```python
from build123d import *

# Parameters (mm, degrees)
F2_SIZE        = 1
F4_D           = 5
F4_DEPTH       = 15
F4_TIP         = 1.5021515476
F7_D           = 9
F7_DEPTH       = 6.3
F7_CSINK_D     = 17.92
F7_CSINK_ANGLE = 90
F7_TIP         = 2.7038727856


with BuildPart() as f1:
    # F0 (on Right) → F1 (revolve)
    with BuildSketch(Plane.YZ):
        Polygon((-17.5, 10), (-17.5, 0), (17.5, 0), (17.5, 10), (9.5, 10), (9.5, 12.5), (7.5, 12.5), (7.5, 10), align=None)
    revolve(axis=Axis((0, 0, 0), (0, 1, 0)))

    # F2
    f2_edges = [f1.edges().sort_by_distance(p)[0] for p in [
        (0, 17.5, -10),
        (0, -17.5, -10),
    ]]
    chamfer(f2_edges, length=F2_SIZE)

    # F4
    with Locations(Plane.XZ.offset(17.5)):
        with Locations((0, 0)):
            Hole(F4_D / 2, depth=F4_DEPTH)
            with Locations((0, 0, -(F4_DEPTH + F4_TIP / 2))):  # 118° drill point
                Cone(0, F4_D / 2, F4_TIP, mode=Mode.SUBTRACT)

    # F7
    with Locations(Plane.XZ.offset(20.5)):
        with Locations((0, 0)):
            CounterSinkHole(F7_D / 2, F7_CSINK_D / 2, depth=F7_DEPTH, counter_sink_angle=F7_CSINK_ANGLE)
            with Locations((0, 0, -(F7_DEPTH + F7_TIP / 2))):  # 118° drill point
                Cone(0, F7_D / 2, F7_TIP, mode=Mode.SUBTRACT)


solid = f1.part
```
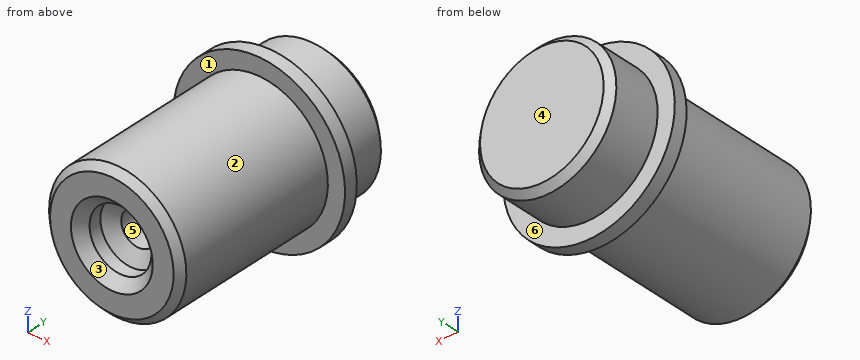
Design review of the part built by this model. Coordinates are the model's own, in mm. Face numbers are marked on the shaded views. A direction names the side the tool comes from. Coordinates: 2 decimals unless noted, no trailing zeros. Order: outer loops, then holes, each group sorted by start corner. A loop starts at its lowest first (then second) coordinate and runs counter-clockwise, first axis right, second up.
1) For the marked faces 4, 5 and 6, list the 3-axis set-ups (+Z, -Z, +X, -X, +Y, -Y) from which the entire face can be reached by the end or side of a thin tool; tool diameter is ignored.
2) Take a section at B-B, the plane y = 15.5. Give the boundary of the cut face in (x, z), and give its area (3 significant figures).
3) Clearance check with flat-ended pins moving along their axes: pin 1 (8 mm diameter, centred on x = 2.5, y = -4, fed in from -Z); pin 2 (2 mm diameter, centred on x = 6.5, z = 9, fed in from -Y); pin 3 (2 mm diameter, centred on x = -2.5, y = -1.5, fed in from +Z). State where each tip first meets the part, or that it passes through.
4) Wall thickness on line 1 along X through (y, z) = (-6.75, 0); line 2 along X through (y, z) = (-15.6, 0); line 3 along Y through (x, z) = (-7.25, -9): over which ranges is each line inside the solid? List them lowest first.
5) Mouldability with a two-part tool opening along X and no side actions: class the marked faces 1, 2 and 3 as +X half, -X half, draft (parallel to the pull), parting line (faces both ways), or undercut.
6) Take a section at A-A, the plane y = -5.5. Give the boundary of the cut face in (x, z).
Returned:
1. face 4: +Z, -Z, +X, -X, +Y
1. face 5: -Y
1. face 6: +Y
2. outline: circle Ø20 at (0, 0)
2. area: 314 mm2
3. pin 1: stops at z = -10
3. pin 2: stops at y = 7.5
3. pin 3: stops at z = 9.89
4. line 1: x = -10 to -2.5, 2.5 to 10
4. line 2: x = -10 to -4.5, 4.5 to 10
4. line 3: y = 7.5 to 9.5
5. face 1: draft
5. face 2: parting line
5. face 3: undercut
6. outline: circle Ø20 at (0, 0); hole circle Ø5 at (0, 0)
